Input: part model. Units: mm. Frame: model coordinates. A direction names the side the tool comes from. Coordinates: 2 decimals unless noted, no trailing zeros. Order: outer loops, then holes, each group sorted by start corner. A loop starts at its lowest first (then second) coordinate and runs counter-clockwise, first axis right, second up. Notation, with made-up numbers: (-11.5, 86.5) -> (17.5, 86.5) arc R10 ccw to (17.5, 103.5) -> close; hole circle Ø4 at (23, 33.25). An arc over 180 degrees is marked (long way). Write each question's results on one line, items separated by ' | '.
```python
from build123d import *

# Parameters (mm, degrees)
F0_W     = 50
F0_H     = 17
F1_DEPTH = 1
F0_W_2   = 52
F0_H_2   = 19
F2_DEPTH = 11
F3_R     = 0.61


with BuildPart() as f1:
    # F0 (on Top) → F1 (new body)
    with BuildSketch(Plane.XY):
        with Locations((6.898358, -7.023614)):
            Rectangle(F0_W, F0_H)
    extrude(amount=F1_DEPTH)

    # F0 (on Top) → F2 (join)
    with BuildSketch(Plane.XY):
        with Locations((6.898358, -7.023614)):
            Rectangle(F0_W_2, F0_H_2)
        with Locations((6.898358, -7.023614)):
            Rectangle(F0_W, F0_H, mode=Mode.SUBTRACT)
    extrude(amount=F2_DEPTH)

    # F3
    f3_edges = [f1.edges().sort_by_distance(p)[0] for p in [
        (6.898358, 1.476386, 1),
        (-18.101642, -7.023614, 1),
        (6.898358, -15.523614, 1),
        (31.898358, -7.023614, 1),
    ]]
    fillet(f3_edges, radius=F3_R)


solid = f1.part
```
(1) Reachability of faces 1 (the face through (31.898, -7, 6)), 2 (the face through (7, 2.476, 5)) from +Z, -Z, +X, -X, +Y, -Y: full face, straight path, thin tool, end or side. Return the list, or none.
Return value:
face 1: +Z | face 2: +Z, -Z, +X, -X, +Y
(2) Cut plane A-A, the plane y = -8.25. Return loops of the section in (x, z).
Return value:
outline: (-19.1, 0) -> (32.9, 0) -> (32.9, 11) -> (31.9, 11) -> (31.9, 1.61) arc R0.61 cw to (31.29, 1) -> (-17.49, 1) arc R0.61 cw to (-18.1, 1.61) -> (-18.1, 11) -> (-19.1, 11) -> close
(3) Cut plane C-C, the plane x = 1. Return loops of the section in (y, z).
Return value:
outline: (-16.52, 0) -> (2.48, 0) -> (2.48, 11) -> (1.48, 11) -> (1.48, 1.61) arc R0.61 cw to (0.87, 1) -> (-14.91, 1) arc R0.61 cw to (-15.52, 1.61) -> (-15.52, 11) -> (-16.52, 11) -> close
(4) Line query: line 1 along Y through (x, z) = (-14.5, 9); line 2 along X through (y, z) = (-1.25, 7); line 3 along Z through (x, y) = (-12, -12). Output: solid intervals per line, ascending. Write a range as from..to.
Return value:
line 1: -16.52..-15.52, 1.48..2.48 | line 2: -19.1..-18.1, 31.9..32.9 | line 3: 0..1
(5) Pin query (flat end, axial travel): P1, Ø10, axis at x = 10, y = -10, coming from the -Z side; P2, Ø8, axis at x = 14, y = -5.5, coming from the +Z side. Return the tip coordinate at first contact, or that it passes through.
Return value:
P1: z = 0 | P2: z = 1
(6) Cut plane B-B, the plane z = 6.75. Return loops of the section in (x, y).
Return value:
outline: (-19.1, -16.52) -> (32.9, -16.52) -> (32.9, 2.48) -> (-19.1, 2.48) -> close; hole (-18.1, -15.52) -> (31.9, -15.52) -> (31.9, 1.48) -> (-18.1, 1.48) -> close
(7) Mould query, pull axis X, two halves, no side actions, for faces 3 (the face through (7, -7, 1)), 4 (the face through (7, -7, 0)), 5 (the face through (-19.102, -7, 5)). Classes: +X half, -X half, draft (parallel to the pull), parting line (faces both ways), or undercut.
Return value:
face 3: undercut | face 4: draft | face 5: -X half
